```python
from build123d import *

# Parameters (mm, degrees)
BOSS_EXTRUDE3_DEPTH              = 2.5
FILLET3_R                        = 2
CUT_EXTRUDE1_DEPTH               = 86.90473786
FILLET1_R                        = 2
FILLET2_R                        = 4
M3_CLEARANCE_HOLE1_D             = 3.4
M3X0_5_TAPPED_HOLE1_D            = 2.5
M3X0_5_TAPPED_HOLE1_DEPTH        = 7.5
M3X0_5_TAPPED_HOLE1_TIP          = 0.751075774
CHAMFER1_SIZE                    = 1
CBORE_FOR_M1_6_SHCS1_D           = 1.8
CBORE_FOR_M1_6_SHCS1_DEPTH       = 5
CBORE_FOR_M1_6_SHCS1_CBORE_D     = 3.5
CBORE_FOR_M1_6_SHCS1_CBORE_DEPTH = 1.6
BOSS_EXTRUDE4_DEPTH              = 5
FILLET4_R                        = 4
M2_CLEARANCE_HOLE1_D             = 2.4
M2_CLEARANCE_HOLE1_DEPTH         = 7.5
M2_CLEARANCE_HOLE1_TIP           = 0.721032743


with BuildPart() as part:
    # Sketch1 → Boss-Extrude3 (new, symmetric)
    with BuildSketch(Plane.XY):
        with BuildLine():
            Line((-39, 0), (-31, 0))
            Line((-31, 0), (-31, 18.037654982))
            Line((-31, 18.037654982), (-21.161883591, 24))
            Line((-21.161883591, 24), (21.161883591, 24))
            Line((21.161883591, 24), (31, 18.037654982))
            Line((31, 18.037654982), (31, 0))
            Line((31, 0), (39, 0))
            Line((39, 0), (39, 20.205165085))
            Line((39, 20.205165085), (24.389646385, 67.734568005))
            ThreePointArc((24.389646385, 67.734568005), (23.767766953, 68.767766953), (22.734568005, 69.389646385))
            Line((22.734568005, 69.389646385), (0, 76.378164175))
            Line((0, 76.378164175), (-22.734568005, 69.389646385))
            ThreePointArc((-22.734568005, 69.389646385), (-23.767766953, 68.767766953), (-24.389646385, 67.734568005))
            Line((-24.389646385, 67.734568005), (-39, 20.205165085))
            Line((-39, 20.205165085), (-39, 0))
        make_face()
        with BuildLine():
            Line((-20, 29), (-20, 43.535898385))
            ThreePointArc((-20, 43.535898385), (-19.171572875, 44.171572875), (-18.535898385, 45))
            Line((-18.535898385, 45), (18.535898385, 45))
            ThreePointArc((18.535898385, 45), (19.171572875, 44.171572875), (20, 43.535898385))
            Line((20, 43.535898385), (20, 29))
            Line((20, 29), (-20, 29))
        make_face(mode=Mode.SUBTRACT)
        with BuildLine():
            Line((18.535898385, 49), (-18.535898385, 49))
            ThreePointArc((-18.535898385, 49), (-22.449787583, 50.974630943), (-25.823434216, 48.175308809))
            Line((-25.823434216, 48.175308809), (-20.719808061, 64.77807629))
            Line((-20.719808061, 64.77807629), (0, 71.147264708))
            Line((0, 71.147264708), (20.719808061, 64.77807629))
            Line((20.719808061, 64.77807629), (25.823434216, 48.175308809))
            ThreePointArc((25.823434216, 48.175308809), (22.449787583, 50.974630943), (18.535898385, 49))
        make_face(mode=Mode.SUBTRACT)
    extrude(amount=BOSS_EXTRUDE3_DEPTH, both=True)

    # Fillet3
    fillet3_edges = [part.edges().sort_by_distance(p)[0] for p in [
        (-18.535898385, 45, 0),
        (-20, 43.535898385, 0),
        (-20, 29, 0),
        (20, 29, 0),
        (20, 43.535898385, 0),
        (18.535898385, 45, 0),
        (20.719808061, 64.77807629, 0),
        (0, 71.147264708, 0),
        (-20.719808061, 64.77807629, 0),
        (-25.823434216, 48.175308809, 0),
        (-18.535898385, 49, 0),
        (18.535898385, 49, 0),
    ]]
    fillet(fillet3_edges, radius=FILLET3_R - 0.0004)  # a hair under: the kernel refuses the full size
    fillet3_2_edges = [part.edges().sort_by_distance(p)[0] for p in [
        (25.823434216, 48.175308809, 0),
    ]]
    fillet(fillet3_2_edges, radius=FILLET3_R)

    # Sketch2 → Cut-Extrude1 (cut, through all)
    with BuildSketch(Plane(origin=(0, 0, -2.5), x_dir=(-1, 0, 0), z_dir=(0, 0, -1))):
        with BuildLine():
            Line((-27.911717108, 41.381849759), (-34.256545, 20.741289696))
            Line((-34.256545, 20.741289696), (-24, 26.957221429))
            Line((-24, 26.957221429), (-24, 40.794195355))
            ThreePointArc((-24, 40.794195355), (-25.702875629, 42.77200149), (-27.911717108, 41.381849759))
        make_face()
        with BuildLine():
            Line((24, 26.957221429), (34.256545, 20.741289696))
            Line((34.256545, 20.741289696), (27.911717108, 41.381849759))
            ThreePointArc((27.911717108, 41.381849759), (25.702875629, 42.77200149), (24, 40.794195355))
            Line((24, 40.794195355), (24, 26.957221429))
        make_face()
    extrude(amount=-CUT_EXTRUDE1_DEPTH, mode=Mode.SUBTRACT)

    # Fillet1
    fillet1_edges = [part.edges().sort_by_distance(p)[0] for p in [
        (24, 26.957221429, 0),
        (34.256545, 20.741289696, 0),
        (-34.256545, 20.741289696, 0),
        (-24, 26.957221429, 0),
    ]]
    fillet(fillet1_edges, radius=FILLET1_R)

    # Fillet2
    fillet2_edges = [part.edges().sort_by_distance(p)[0] for p in [
        (39, 20.205165085, 0),
        (31, 18.037654982, 0),
        (21.161883591, 24, 0),
        (-21.161883591, 24, 0),
        (-31, 18.037654982, 0),
        (-39, 20.205165085, 0),
        (0, 76.378164175, 0),
    ]]
    fillet(fillet2_edges, radius=FILLET2_R)

    # M3 Clearance Hole1 (through all)
    with Locations(Plane.XY.offset(2.5)):
        with Locations((-22, 47), (22, 47)):
            Hole(M3_CLEARANCE_HOLE1_D / 2)

    # M3x0.5 Tapped Hole1
    with Locations(Plane(origin=(0, 0, 0), x_dir=(-1, 0, 0), z_dir=(0, -1, 0))):
        with Locations((-35, 0), (35, 0)):
            Hole(M3X0_5_TAPPED_HOLE1_D / 2, depth=M3X0_5_TAPPED_HOLE1_DEPTH)
            with Locations((0, 0, -(M3X0_5_TAPPED_HOLE1_DEPTH + M3X0_5_TAPPED_HOLE1_TIP / 2))):  # 118° drill point
                Cone(0, M3X0_5_TAPPED_HOLE1_D / 2, M3X0_5_TAPPED_HOLE1_TIP, mode=Mode.SUBTRACT)

    # Chamfer1
    chamfer1_edges = [part.edges().sort_by_distance(p)[0] for p in [
        (39, 0, 0),
        (31, 0, 0),
        (-31, 0, 0),
        (-39, 0, 0),
    ]]
    chamfer(chamfer1_edges, length=CHAMFER1_SIZE)

    # CBORE for M1.6 SHCS1
    with Locations(Plane(origin=(0, 24, 0), x_dir=(-1, 0, 0), z_dir=(0, -1, 0))):
        with Locations((12.75, 0), (-12.75, 0)):
            CounterBoreHole(CBORE_FOR_M1_6_SHCS1_D / 2, CBORE_FOR_M1_6_SHCS1_CBORE_D / 2, CBORE_FOR_M1_6_SHCS1_CBORE_DEPTH, depth=CBORE_FOR_M1_6_SHCS1_DEPTH)

    # Sketch12 → Boss-Extrude4 (add)
    with BuildSketch(Plane.XY.offset(2.5)):
        with BuildLine():
            Line((-41.503743829, 31.294305745), (-38.062285211, 36.209218011))
            ThreePointArc((-38.062285211, 36.209218011), (-32.491371289, 37.191520443), (-31.509068857, 31.62060652))
            Line((-31.509068857, 31.62060652), (-34.950527475, 26.705694255))
            ThreePointArc((-34.950527475, 26.705694255), (-40.521441398, 25.723391823), (-41.503743829, 31.294305745))
        make_face()
    extrude(amount=-BOSS_EXTRUDE4_DEPTH)

    # Fillet4
    fillet4_edges = [part.edges().sort_by_distance(p)[0] for p in [
        (-33.610368225, 37.738346482, 0),
        (-37.505935548, 25.065553354, 0),
    ]]
    fillet(fillet4_edges, radius=FILLET4_R)

    # M2 Clearance Hole1
    with Locations(Plane.XY.offset(2.5)):
        with Locations((-38.227135652, 29), (-34.785677034, 33.914912266)):
            Hole(M2_CLEARANCE_HOLE1_D / 2, depth=M2_CLEARANCE_HOLE1_DEPTH)
            with Locations((0, 0, -(M2_CLEARANCE_HOLE1_DEPTH + M2_CLEARANCE_HOLE1_TIP / 2))):  # 118° drill point
                Cone(0, M2_CLEARANCE_HOLE1_D / 2, M2_CLEARANCE_HOLE1_TIP, mode=Mode.SUBTRACT)


solid = part.part
```
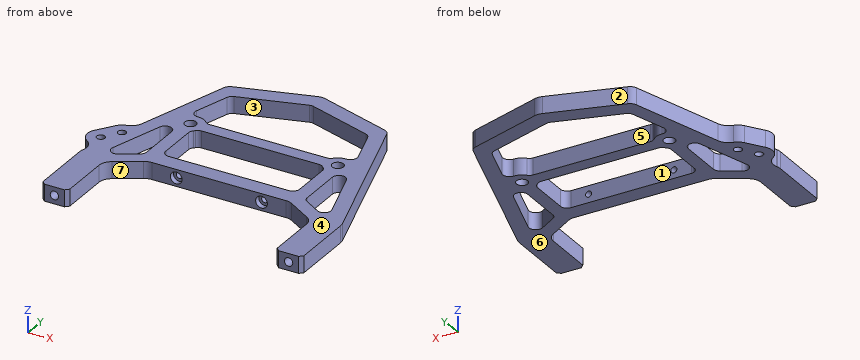
Read the model definition and answer for the solid it produces. Units are mm, in the model's axes. Face numbers are marked on the shaded views. A direction names the side the tool comes from. Coordinates: 2 decimals unless noted, no trailing zeros. Loops run counter-clockwise (first coordinate to the right, second up) from the corner with the lowest first, then second, coordinate; pieces in that order, holes last. Notation, with made-up numbers: (-25, 31) - (9, 31) arc R23 ccw to (9, 54) - close; hole circle Ø10 at (-30, 38). An arc over 180 degrees is marked (long way). Answer in a Markdown table with one row per item.
1. Find section D-D, the plane x = 12.75. Write down the section's boundary in (y, z).
Conclusion:
| item | result |
|---|---|
| outline | (24, -2.5) - (29, -2.5) - (29, -0.9) - (25.6, -0.9) - (25.6, -1.75) - (24, -1.75) - close; (24, 1.75) - (25.6, 1.75) - (25.6, 0.9) - (29, 0.9) - (29, 2.5) - (24, 2.5) - close; (45, -2.5) - (49, -2.5) - (49, 2.5) - (45, 2.5) - close; (67.23, -2.5) - (72.46, -2.5) - (72.46, 2.5) - (67.23, 2.5) - close |
2. Which of the six approach directions +Z, -Z, +X, -X, +Y, -Y give full straight-line access (tool end or side, diameter ignored) to the marked faces 5, 6 and 7?
Conclusion:
| item | result |
|---|---|
| face 5 | +Z, -Z |
| face 6 | -Z, +X, -X, +Y, -Y |
| face 7 | +Z, -Z, -Y |
3. Find section A-A, the plane y = 6. Write down the section's boundary in (x, z), then the cut area to 3 significant figures.
Conclusion:
| item | result |
|---|---|
| outline | (-39, -2.5) - (-31, -2.5) - (-31, 2.5) - (-39, 2.5) - close; (31, -2.5) - (39, -2.5) - (39, 2.5) - (31, 2.5) - close; hole circle Ø2.5 at (-35, 0); hole circle Ø2.5 at (35, 0) |
| area | 70.2 mm² |
4. Given pin 1 (3 mm diameter, centred on x = -12.75, z = 0, fed in from -Y); pin 2 (1 mm diameter, centred on y = 20.5, z = 0, fed in from +X); pin 3 (1.5 mm diameter, centred on x = 8.5, z = 1, fed in from -Y), each flat-ended and moving along its own axis, determine where each tip first touches the part or whether it passes through.
Conclusion:
| item | result |
|---|---|
| pin 1 | stops at y = 25.6 |
| pin 2 | stops at x = 38.98 |
| pin 3 | stops at y = 24 |
5. Straight lines are drawn through the part: line 1 (X direction, y = 12.5, z = -1.7); line 2 (Y direction, x = -2, z = -0.95); line 3 (Y direction, x = 12, z = 1.2). For each, find the intervals that lie inside material, in ascending order.
Conclusion:
| item | result |
|---|---|
| line 1 | x = -39 to -31, 31 to 39 |
| line 2 | y = 24 to 29, 45 to 49, 70.53 to 75.76 |
| line 3 | y = 25.6 to 29, 45 to 49, 67.46 to 72.69 |
6. Find section C-C, the plane y = 47. Write down the section's boundary in (x, z), then the cut area to 3 significant figures.
Conclusion:
| item | result |
|---|---|
| outline | (-30.76, -2.5) - (-23.7, -2.5) - (-23.7, 2.5) - (-30.76, 2.5) - close; (-20.3, -2.5) - (20.3, -2.5) - (20.3, 2.5) - (-20.3, 2.5) - close; (23.7, -2.5) - (30.76, -2.5) - (30.76, 2.5) - (23.7, 2.5) - close |
| area | 274 mm² |
7. Determine the mould class of the marked faces 1, 2, 3 and 4 for opening direction Y: +Y half, -Y half, draft (parallel to the pull), parting line (faces both ways), or undercut.
Conclusion:
| item | result |
|---|---|
| face 1 | undercut |
| face 2 | +Y half |
| face 3 | undercut |
| face 4 | draft |
8. Find section B-B, the plane x = -10. Write down the section's boundary in (y, z), then the cut area to 3 significant figures.
Conclusion:
| item | result |
|---|---|
| outline | (24, -2.5) - (29, -2.5) - (29, 2.5) - (24, 2.5) - close; (45, -2.5) - (49, -2.5) - (49, 2.5) - (45, 2.5) - close; (68.07, -2.5) - (73.3, -2.5) - (73.3, 2.5) - (68.07, 2.5) - close |
| area | 71.2 mm² |
